Verification items for this drawing (mm, ordinates from the low corner). Coordinates: 2 decimals unless noted, no trailing zeros. Write each loop counter-clockwise with the first axis right and the second up, starting at its lowest first coordinate (ties: lowest second). Pieces come first, ordered by that corner, then holes. Notation, with made-up numbers: (29, 69) -> (78, 69) arc R16 cw to (78, 79) -> close; hole circle Ø1 at (51, 10.5). An arc over 180 degrees is marked (long way). Use CSV: the item, a comma, the result in double quotes.
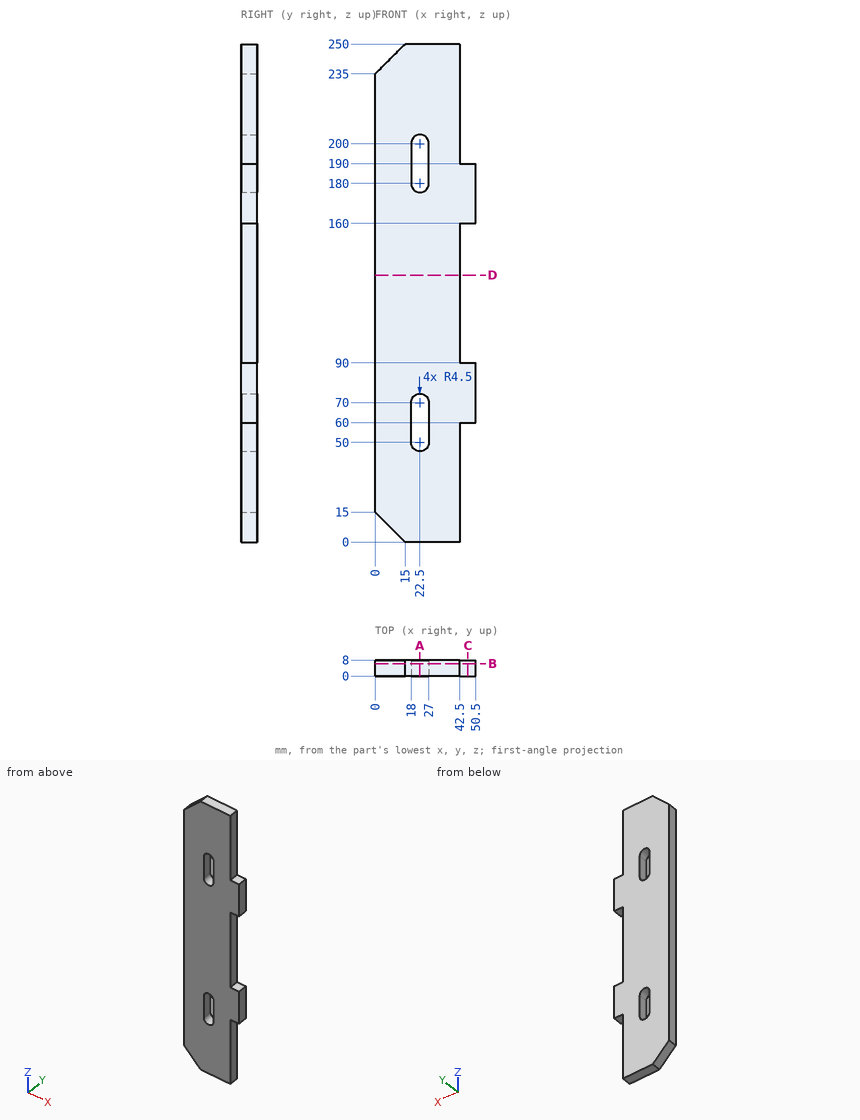
1) Gauge pin test, flat ends, axial feed: pin 1 (2.5 mm diameter, centred on y = 4.5, z = 41, fed in from +X); pin 2 (1.5 mm diameter, centred on x = 6.5, y = 2, fed in from -Z); pin 3 (2.5 mm diameter, centred on x = 45, y = 3.5, fed in from +Z). Record the tip position at first contact, or that the pin passes through.
Return value:
pin 1,"x = 42.5"
pin 2,"z = 7.75"
pin 3,"z = 190"
2) Scan lines: L1, parallel to Z at x = 21, y = 3; L2, parallel to X at y = 5, z = 57; L3, parallel to X at y = 6, z = 69.5. Record each from-to range of solid material in increasing order.
Return value:
L1,"0 to 45.76, 74.24 to 175.76, 204.24 to 250"
L2,"0 to 18, 27 to 42.5"
L3,"0 to 18, 27 to 50.5"
3) Cross-section at D-D (z = 134). Record the boundary of the cut face in (x, y), plus the area to 3 significant figures.
Return value:
outline,"(0, 0) -> (42.5, 0) -> (42.5, 8) -> (0, 8) -> close"
area,"340 mm2"
4) Cross-section at A-A (x = 22.5). Record the boundary of the cut face in (y, z).
Return value:
outline,"(0, 0) -> (8, 0) -> (8, 45.5) -> (0, 45.5) -> close; (0, 74.5) -> (8, 74.5) -> (8, 175.5) -> (0, 175.5) -> close; (0, 204.5) -> (8, 204.5) -> (8, 250) -> (0, 250) -> close"
5) Cross-section at C-C (x = 46.5). Record the boundary of the cut face in (y, z), plus the area to 3 significant figures.
Return value:
outline,"(0, 60) -> (8, 60) -> (8, 90) -> (0, 90) -> close; (0, 160) -> (8, 160) -> (8, 190) -> (0, 190) -> close"
area,"480 mm2"
6) Cross-section at B-B (y = 6.25). Record the boundary of the cut face in (x, z).
Return value:
outline,"(0, 15) -> (15, 0) -> (42.5, 0) -> (42.5, 60) -> (50.5, 60) -> (50.5, 90) -> (42.5, 90) -> (42.5, 160) -> (50.5, 160) -> (50.5, 190) -> (42.5, 190) -> (42.5, 250) -> (15, 250) -> (0, 235) -> close; hole (18, 50) arc R4.5 ccw to (27, 50) -> (27, 70) arc R4.5 ccw to (18, 70) -> close; hole (18, 180) arc R4.5 ccw to (27, 180) -> (27, 200) arc R4.5 ccw to (18, 200) -> close"
